Design review of the part built by this model. Coordinates are the model's own, in mm. Face numbers are marked on the shaded views. A direction names the side the tool comes from. Round coordinates to 2 decimals unless told otherwise and drop trailing zeros. Loops run counter-clockwise (first coordinate to the right, second up) from the corner with the lowest first, then second, coordinate; pieces in that order, holes last. Notation, with made-up numbers: (0.25, -30.75) - (41.25, -30.75) arc R18 ccw to (41.25, -12.75) - close; hole circle Ø6 at (38.25, -32.5). An arc over 180 degrees is marked (long way). Use one line per item in the form item = value. Start each with the question number.
(1) Machinability: for the marked faces 1 and 2, which of the approach directions +Z, -Z, +X, -X, +Y, -Y give a long, thin tool a straight path to every point of the face, cutting with its end or side? Answer none if there is none.
(2) The part is to be moulded in two halves that separate along Z. For the marked faces 3, 4 and 5, say which applies: released by +Z, released by -Z, zero draft, split by the parting line, or undercut.
(3) We need section C-C, the plane z = -0.75. Write out the cut boundary in (x, y).
(4) We need section D-D, the plane x = -9.25. Write out the cut boundary in (y, z), then the cut area to 3 significant figures.
(5) We need section A-A, the plane y = -1.15. Write out the cut boundary in (x, z), then the cut area to 3 significant figures.
(6) Wall thickness on probe 1 along X at (y, z) = (-2.45, 1.5); probe 2 along Z at (x, y) = (-2.5, -2.1); probe 3 along X at (y, z) = (-2.45, -3): over which ranges is each line inside the solid? List them lowest first. Write a range as [from, to].
(7) For pin 1 (1 mm diameter, centred on y = -1, z = -4, fed in from +X); pin 2 (1.5 mm diameter, centred on x = -8.5, y = -2, fed in from -Z), all flat-tipped, find the tip position at first contact; note any pin that passes through.
(8) We need section B-B, the plane z = 0.5. Write out the cut boundary in (x, y), then the cut area to 3 significant figures.
from build123d import *

# Parameters (mm, degrees)
PAD_DEPTH = 2.65


with BuildPart() as part:
    # Sketch → Pad (new body)
    with BuildSketch(Plane.XZ):
        with BuildLine():
            ThreePointArc((-6.45, 6.05), (-12.5, 0), (-6.45, -6.05))
            Line((-6.45, -6.05), (6.45, -6.05))
            ThreePointArc((6.45, -6.05), (12.5, 0), (6.45, 6.05))
            Line((6.45, 6.05), (-6.45, 6.05))
        make_face()
        Polygon((1.760918, 3.05), (-1.760918, 3.05), (-3.521837, 0), (-1.760918, -3.05), (1.760918, -3.05), (3.521837, 0), align=None, mode=Mode.SUBTRACT)
    extrude(amount=PAD_DEPTH)


solid = part.part
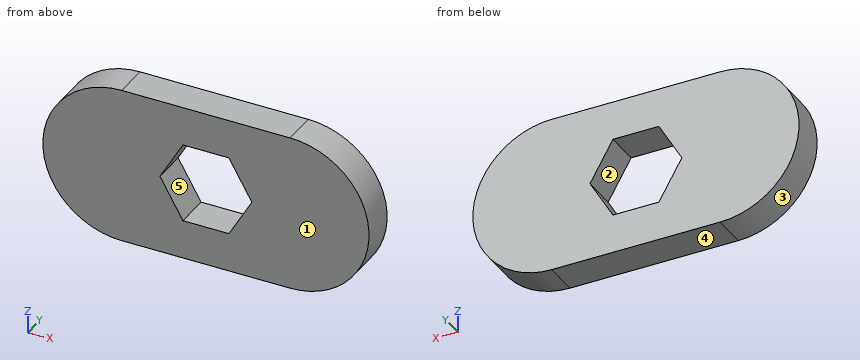
Data:
q1.face_1 = +Z, -Z, +X, -X, -Y
q1.face_2 = +Y, -Y
q2.face_3 = split by the parting line
q2.face_4 = released by -Z
q2.face_5 = undercut
q3.outline = (-12.45, -2.65) - (-3.09, -2.65) - (-3.09, 0) - (-12.45, 0) - close; (3.09, -2.65) - (12.45, -2.65) - (12.45, 0) - (3.09, 0) - close
q4.outline = (-2.65, -5.36) - (0, -5.36) - (0, 5.36) - (-2.65, 5.36) - close
q4.area = 28.4 mm^2
q5.outline = (-6.45, -6.05) - (6.45, -6.05) arc R6.05 ccw to (6.45, 6.05) - (-6.45, 6.05) arc R6.05 ccw to start; hole (-3.52, 0) - (-1.76, -3.05) - (1.76, -3.05) - (3.52, 0) - (1.76, 3.05) - (-1.76, 3.05) - close
q5.area = 239 mm^2
q6.probe_1 = [-12.31, -2.66], [2.66, 12.31]
q6.probe_2 = [-6.05, -1.77], [1.77, 6.05]
q6.probe_3 = [-11.7, -1.79], [1.79, 11.7]
q7.pin_1 = 11.38
q7.pin_2 = -5.91
q8.outline = (-12.48, -2.65) - (-3.23, -2.65) - (-3.23, 0) - (-12.48, 0) - close; (3.23, -2.65) - (12.48, -2.65) - (12.48, 0) - (3.23, 0) - close
q8.area = 49.0 mm^2
